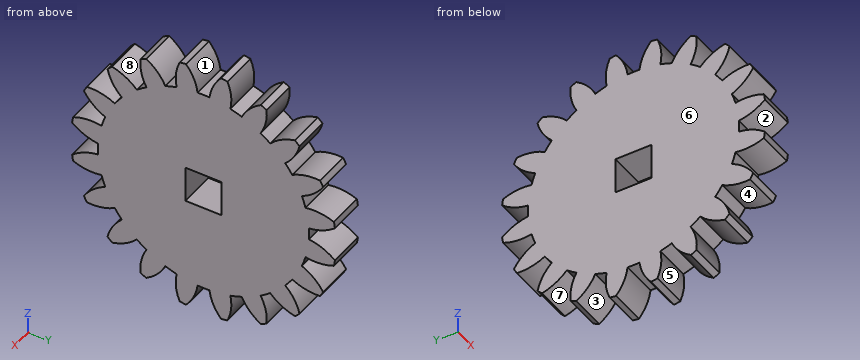
from build123d import *

# Parameters (mm, degrees)
BASPROSKE_W           = 6
BASPROSKE_H           = 22
TOOTHCUT_DEPTH        = 32.685959036
TEETHCUTS_COUNT       = 20
TEETHCUTS_ANGLE       = 342
BORSKE_R              = 0.5
BORE_DEPTH            = 50.0000508
CORTAR_EXTRUIR1_DEPTH = 10


with BuildPart() as part:
    # BasProSke → Base-Revolve (revolve)
    with BuildSketch(Plane(origin=(0, 0, 0), x_dir=(1, 0, 0), z_dir=(0, 1, 0)), mode=Mode.PRIVATE) as base_revolve_sk:
        with Locations((3, 11)):
            Rectangle(BASPROSKE_W, BASPROSKE_H)
    revolve(base_revolve_sk.sketch.rotate(Axis((-10, 0, 0), (1, 0, 0)), 180), axis=Axis((-10, 0, 0), (1, 0, 0)))

    # TooCutSke → ToothCut (cut, through all)
    with BuildSketch(Plane(origin=(0, 0, 0), x_dir=(0, 0, -1), z_dir=(1, 0, 0))):
        with BuildLine():
            ThreePointArc((0.986171591, 17.471189616), (0, 17.499), (-0.986171591, 17.471189616))
            ThreePointArc((-0.986171591, 17.471189616), (-1.626916196, 19.798789858), (-2.932850173, 21.829260982))
            ThreePointArc((-2.932850173, 21.829260982), (0, 22.0254), (2.932850173, 21.829260982))
            ThreePointArc((2.932850173, 21.829260982), (1.626916196, 19.798789858), (0.986171591, 17.471189616))
        make_face()
    toothcut = extrude(amount=TOOTHCUT_DEPTH, mode=Mode.SUBTRACT)

    # TeethCuts: ToothCut ×20 about axis
    teethcuts_axis = Axis((-10, 0, 0), (1, 0, 0))
    for i in range(1, TEETHCUTS_COUNT):
        add(toothcut.rotate(teethcuts_axis, i * TEETHCUTS_ANGLE / (TEETHCUTS_COUNT - 1)), mode=Mode.SUBTRACT)

    # BorSke → Bore (cut, symmetric)
    with BuildSketch(Plane(origin=(0, 0, 0), x_dir=(0, 0, -1), z_dir=(1, 0, 0))):
        with Locations(Location((0, 0, 0), (0, 0, 180))):
            Circle(BORSKE_R)
    extrude(amount=BORE_DEPTH, both=True, mode=Mode.SUBTRACT)

    # Croquis1 → Cortar-Extruir1 (cut)
    with BuildSketch(Plane(origin=(6, 0, 0), x_dir=(0, 0, -1), z_dir=(1, 0, 0))):
        Polygon((0, 3), (-3, 3), (-3, -3), (3, -3), (3, 3), align=None)
    extrude(amount=-CORTAR_EXTRUIR1_DEPTH, mode=Mode.SUBTRACT)


solid = part.part
The model under review builds one solid part; all positions refer to its coordinate system, in mm. Face numbers are marked on the shaded views. A direction names the side the tool comes from. Round coordinates to 2 decimals unless told otherwise and drop trailing zeros. Write each loop counter-clockwise with the first axis right and the second up, starting at its lowest first coordinate (ties: lowest second). Pieces come first, ordered by that corner, then holes. Notation, with made-up numbers: (41, 43) - (71, 43) arc R35 cw to (71, 80) - close; hole circle Ø4 at (67, 77.25). An arc over 180 degrees is marked (long way). One line per item, written item: value. Start each with the question number.
1. Consider section C-C on z = -8. Write out the cut boundary in (x, y).
2. The part is to be moulded in two halves that separate along Z. For the marked faces 5, 6, 7 and 8, say which applies: released by +Z, released by -Z, zero draft, split by the parting line, or undercut.
3. Clearance check with flat-ended pins moving along their axes: P1, Ø3, axis at x = 4, y = -5, coming from the +Z side; P2, Ø1.5, axis at x = 0.5, z = 11.5, coming from the -Y side; P3, Ø3, axis at x = 4, z = 6.5, coming from the -Y side. State where each tip first meets the part, or that it passes through.
4. Consider section A-A on z = 0. Write out the cut boundary in (x, y).
5. Consider section B-B on y = 13. Write out the cut boundary in (x, z), and give its area (3 significant figures).
6. To check wall thickness, follow L1, parallel to Z at x = 5.05, y = -17; L2, parallel to Y at x = 1.3, z = 18; L3, parallel to Y at x = 3.05, z = 14.5. State the ranges of each line that lie inside material, in increasing order. Write a range as from..to.
7. Machinability: for the marked faces 1, 2, 3 and 4, which of the approach directions +Z, -Z, +X, -X, +Y, -Y give a long, thin tool a straight path to every point of the face, cutting with its end or side? Answer none if there is none.
Checks:
1. outline: (0, -18.68) - (6, -18.68) - (6, 18.68) - (0, 18.68) - close
2. face 5: undercut
2. face 6: zero draft
2. face 7: released by -Z
2. face 8: released by +Z
3. P1: stops at z = 21.72
3. P2: stops at y = -14.61
3. P3: stops at y = -18.68
4. outline: (0, -17.5) - (6, -17.5) - (6, -3) - (0, -3) - close; (0, 3) - (6, 3) - (6, 17.5) - (0, 17.5) - close
5. outline: (0, -15.09) - (6, -15.09) - (6, 15.09) - (0, 15.09) - close
5. area: 181 mm^2
6. L1: z = -10.33..-6.7, -4.48..4.48, 6.7..10.33
6. L2: y = -10.47..-7.39, -4.6..-1.07, 1.07..4.6, 7.39..10.47
6. L3: y = -15.75..-12.11, -9.8..9.8, 12.11..15.75
7. face 1: +Z, +X, -X
7. face 2: +X, -X, -Y
7. face 3: -Z, +X, -X
7. face 4: +X, -X
